The model under review builds one solid part; all positions refer to its coordinate system, in mm. Face numbers are marked on the shaded views. A direction names the side the tool comes from. Round coordinates to 2 decimals unless told otherwise and drop trailing zeros. Order: outer loops, then holes, each group sorted by start corner. A loop starts at its lowest first (then second) coordinate and runs counter-clockwise, first axis right, second up.
1) To check wall thickness, follow L1, parallel to Y at x = 57.5, z = 57; L2, parallel to X at y = 34, z = -45; L3, parallel to Z at x = 29, y = 10.5. State the ranges of each line that lie inside material, in increasing order.
2) Consider section D-D (x = 117). Give the boundary of the cut face in (y, z), then the cut area to 3 significant figures.
3) Consider section B-B (x = 35). Give the boundary of the cut face in (y, z), then the cut area to 3 significant figures.
4) Mouldability with a two-part tool opening along X and no side actions: class the marked faces 3, 4, 5 and 6 as pulls with the +X half, pulls with the -X half, needs draft (parallel to the pull), parting line crosses it, or undercut.
5) Consider section C-C (z = 12). Give the boundary of the cut face in (x, y) (3 decimals), then the cut area to 3 significant figures.
6) Clearance check with flat-ended pins moving along their axes: P1, Ø1, axis at y = 20, z = -2.5, coming from the +X side; P2, Ø5.5, axis at x = 169.5, z = 35.66, coming from the -Y side (3 decimals); P3, Ø6, axis at x = 121.5, y = 36.5, coming from the +Z side. State where each tip first meets the part, or that it passes through.
7) Machinability: for the marked faces 1 and 2, which of the approach directions +Z, -Z, +X, -X, +Y, -Y give a long, thin tool a straight path to every point of the face, cutting with its end or side? Answer none if there is none.
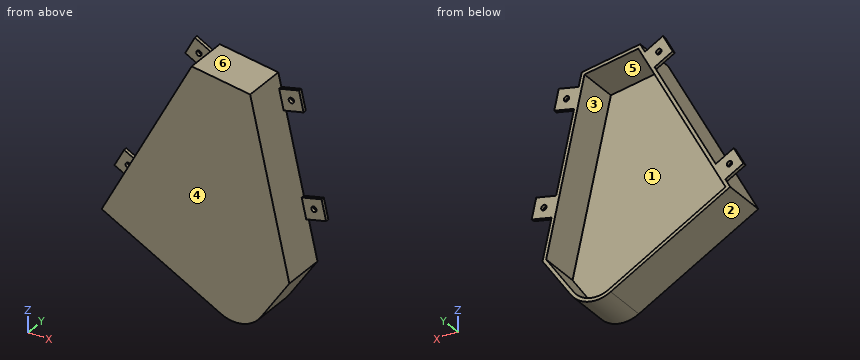
from build123d import *

# Parameters (mm, degrees)
BOSS_EXTRUDE1_DEPTH      = 2.54
BOSS_EXTRUDE5_DEPTH      = 38.1
BOSS_EXTRUDE5_DEPTH_BACK = 2.54
SKETCH6_W                = 19.05
SKETCH6_H                = 3.175
BOSS_EXTRUDE6_DEPTH      = 19.05
SKETCH7_W                = 19.05
SKETCH7_H                = 3.175
BOSS_EXTRUDE7_DEPTH      = 19.05
CUT_EXTRUDE2_REACH       = 5.175
SKETCH8_R                = 2.4892


with BuildPart() as part:
    # Sketch1 → Boss-Extrude1 (new body)
    with BuildSketch(Plane(origin=(0, 0, 0), x_dir=(1, 0, 0), z_dir=(0, 1, 0))):
        with BuildLine():
            Line((108.694500094, 58.18760289), (0, 0))
            Line((0, 0), (81.435616874, -152.121813345))
            Line((81.435616874, -152.121813345), (131.633654365, -144.676094857))
            Line((131.633654365, -144.676094857), (167.396796738, 12.253350144))
            Line((167.396796738, 12.253350144), (141.688668345, 50.073487268))
            ThreePointArc((141.688668345, 50.073487268), (126.748044303, 60.459528823), (108.694500094, 58.18760289))
        make_face()
    extrude(amount=BOSS_EXTRUDE1_DEPTH)

    # Sketch2 → Boss-Extrude5 (add, two sides)
    with BuildSketch(Plane(origin=(0, 2.54, 0), x_dir=(1, 0, 0), z_dir=(0, 1, 0))) as boss_extrude5_sk:
        with BuildLine():
            Line((79.691089457, -155.590310016), (-4.297615284, 1.300674006))
            Line((-4.297615284, 1.300674006), (107.196029455, 60.986747535))
            ThreePointArc((107.196029455, 60.986747535), (127.50626669, 63.54266421), (144.314468737, 51.85836746))
            Line((144.314468737, 51.85836746), (170.799497483, 12.895304744))
            Line((170.799497483, 12.895304744), (134.24691646, -147.498214188))
            Line((134.24691646, -147.498214188), (79.691089457, -155.590310016))
        make_face()
        with BuildLine():
            Line((81.435616874, -152.121813345), (0, 0))
            Line((0, 0), (108.694500094, 58.18760289))
            ThreePointArc((108.694500094, 58.18760289), (126.748044303, 60.459528823), (141.688668345, 50.073487268))
            Line((141.688668345, 50.073487268), (167.396796738, 12.253350144))
            Line((167.396796738, 12.253350144), (131.633654365, -144.676094857))
            Line((131.633654365, -144.676094857), (81.435616874, -152.121813345))
        make_face(mode=Mode.SUBTRACT)
    extrude(amount=BOSS_EXTRUDE5_DEPTH)
    extrude(boss_extrude5_sk.sketch, amount=-BOSS_EXTRUDE5_DEPTH_BACK)

    # Sketch6 → Boss-Extrude6 (add)
    with BuildSketch(Plane(origin=(159.573264194, 0, 36.365650604), x_dir=(0.222196249, 0, -0.975001963), z_dir=(0.975001963, 0, 0.222196249))):
        with Locations((2.898955068, 39.0525)):
            Rectangle(SKETCH6_W, SKETCH6_H)
        with Locations((-91.756887063, 39.0525)):
            Rectangle(SKETCH6_W, SKETCH6_H)
    extrude(amount=BOSS_EXTRUDE6_DEPTH)

    # Sketch7 → Boss-Extrude7 (add)
    with BuildSketch(Plane(origin=(-2.799144645, 0, 1.498470639), x_dir=(0.471959256, 0, 0.881620361), z_dir=(-0.881620361, 0, 0.471959256))):
        with Locations((15.875, 39.0525)):
            Rectangle(SKETCH7_W, SKETCH7_H)
        with Locations((155.73253255, 39.0525)):
            Rectangle(SKETCH7_W, SKETCH7_H)
    extrude(amount=BOSS_EXTRUDE7_DEPTH)

    # Sketch8 → Cut-Extrude2 (cut, up to next)
    with BuildSketch(Plane(origin=(0, 37.465, 0), x_dir=(-1, 0, 0), z_dir=(0, -1, 0)), mode=Mode.PRIVATE) as cut_extrude2_sk1:
        with Locations((3.704225384, -19.989605782)):
            Circle(SKETCH8_R)
    cut_extrude2_tool1 = extrude(cut_extrude2_sk1.sketch, amount=-CUT_EXTRUDE2_REACH, mode=Mode.PRIVATE) & part.part
    add(cut_extrude2_tool1.solids().sort_by_distance((-3.704225, 37.465, 19.989606))[0], mode=Mode.SUBTRACT)
    # Sketch8 → Cut-Extrude2 (cut, up to next)
    with BuildSketch(Plane(origin=(0, 37.465, 0), x_dir=(-1, 0, 0), z_dir=(0, -1, 0)), mode=Mode.PRIVATE) as cut_extrude2_sk2:
        with Locations((-62.302831686, -143.290854064)):
            Circle(SKETCH8_R)
    cut_extrude2_tool2 = extrude(cut_extrude2_sk2.sketch, amount=-CUT_EXTRUDE2_REACH, mode=Mode.PRIVATE) & part.part
    add(cut_extrude2_tool2.solids().sort_by_distance((62.302832, 37.465, 143.290854))[0], mode=Mode.SUBTRACT)
    # Sketch8 → Cut-Extrude2 (cut, up to next)
    with BuildSketch(Plane(origin=(0, 37.465, 0), x_dir=(-1, 0, 0), z_dir=(0, -1, 0)), mode=Mode.PRIVATE) as cut_extrude2_sk3:
        with Locations((-148.472121782, -127.945214839)):
            Circle(SKETCH8_R)
    cut_extrude2_tool3 = extrude(cut_extrude2_sk3.sketch, amount=-CUT_EXTRUDE2_REACH, mode=Mode.PRIVATE) & part.part
    add(cut_extrude2_tool3.solids().sort_by_distance((148.472122, 37.465, 127.945215))[0], mode=Mode.SUBTRACT)
    # Sketch8 → Cut-Extrude2 (cut, up to next)
    with BuildSketch(Plane(origin=(0, 37.465, 0), x_dir=(-1, 0, 0), z_dir=(0, -1, 0)), mode=Mode.PRIVATE) as cut_extrude2_sk4:
        with Locations((-169.504294829, -35.655582993)):
            Circle(SKETCH8_R)
    cut_extrude2_tool4 = extrude(cut_extrude2_sk4.sketch, amount=-CUT_EXTRUDE2_REACH, mode=Mode.PRIVATE) & part.part
    add(cut_extrude2_tool4.solids().sort_by_distance((169.504295, 37.465, 35.655583))[0], mode=Mode.SUBTRACT)


solid = part.part
Answer below:
1. L1: y = 0 to 2.54
1. L2: x = 77.33 to 84.06, 145.14 to 148.98
1. L3: z = -19.13 to -15.52, 54.17 to 60.9
2. outline: (0, -64.13) - (40.64, -64.13) - (40.64, -60.93) - (2.54, -60.93) - (2.54, 146.85) - (40.64, 146.85) - (40.64, 150.06) - (0, 150.06) - close
2. area: 788 mm2
3. outline: (0, -22.34) - (40.64, -22.34) - (40.64, -18.74) - (2.54, -18.74) - (2.54, 65.38) - (40.64, 65.38) - (40.64, 72.11) - (0, 72.11) - close
3. area: 633 mm2
4. face 3: undercut
4. face 4: needs draft
4. face 5: undercut
4. face 6: pulls with the +X half
5. outline: (-8.961, 37.465) - (2.823, 37.465) - (2.823, 0) - (165.126, 0) - (165.126, 40.64) - (161.87, 40.64) - (161.87, 2.54) - (6.424, 2.54) - (6.424, 40.64) - (-8.961, 40.64) - close
5. area: 711 mm2
6. P1: stops at x = 168.54
6. P2: stops at y = 37.465
6. P3: stops at z = 149.83
7. face 1: +Y
7. face 2: -Z, -X, +Y, -Y
